Geometry: final body of the model. Coordinates: model frame, mm. Face numbers are marked on the shaded views. A direction names the side the tool comes from. Give positions to 0.01 mm unless a question says otherwise; leave off trailing zeros. Order: outer loops, then holes, each group sorted by start corner. A loop starts at its lowest first (then second) coordinate and runs counter-clockwise, first axis right, second up. Notation, with made-up numbers: (51, 65) -> (66, 65) arc R7 ccw to (66, 72) -> close; hole circle Ø1 at (-22.5, -19). An arc over 180 degrees is marked (long way). Write item = value, one per line.
```python
from build123d import *

# Parameters (mm, degrees)
SKETCH1_W                = 40
SKETCH1_H                = 48
BOSS_EXTRUDE1_DEPTH      = 4
BOSS_EXTRUDE2_DEPTH      = 11.15
BOSS_EXTRUDE2_DEPTH_BACK = 4
SKETCH5_W                = 40
SKETCH5_H                = 5.225
SKETCH5_W_2              = 18
SKETCH5_H_2              = 5
SKETCH5_H_3              = 6
FILLET1_DEPTH            = 40
SKETCH6_R                = 1.35
CUT_EXTRUDE4_DEPTH       = 58.214705278
CHAMFER2_SIZE            = 2
CHAMFER3_SIZE            = 3
CHAMFER3_SIZE2           = 1
CHAMFER4_SIZE            = 3
CHAMFER4_SIZE2           = 0.5
CUT_EXTRUDE6_DEPTH       = 10
CUT_EXTRUDE6_DEPTH_BACK  = 10
CUT_EXTRUDE8_REACH       = 66.292
SKETCH12_R               = 3
SKETCH13_R               = 1.5
CUT_EXTRUDE10_DEPTH      = 10.275
CUT_EXTRUDE7_DEPTH       = 1.25
CUT_EXTRUDE7_DEPTH_BACK  = 1.25
CHAMFER5_SIZE            = 5
CHAMFER5_SIZE2           = 3
CHAMFER6_SIZE            = 3
CHAMFER6_SIZE2           = 5
CUT_EXTRUDE12_DEPTH      = 46.535947422
CUT_EXTRUDE12_DEPTH_BACK = 46.535947422
SKETCH15_R               = 3.5


with BuildPart() as part:
    # Sketch1 → Boss-Extrude1 (new body)
    with BuildSketch(Plane.XY):
        with Locations((20, 14)):
            Rectangle(SKETCH1_W, SKETCH1_H)
    extrude(amount=BOSS_EXTRUDE1_DEPTH)

    # Sketch5 → Boss-Extrude2 (add, two sides: drawn at the far end of the back side and taken through both)
    with BuildSketch(Plane.XY.offset(4).offset(-BOSS_EXTRUDE2_DEPTH_BACK)):
        Polygon((0.9, 8.125), (0, 8.125), (0, 15.5), (40, 15.5), (40, 9), (28, 9), (27.357142857, 10.5), (11.081237185, 10.5), (9.763380042, 7.425), (8.800403155, 7.425), (8.500403155, 8.125), (7.531690021, 8.125), (7.231690021, 7.425), (6.221941609, 7.425), (5.921941609, 8.125), (5, 8.125), (4.7, 7.425), (3.7, 7.425), (3.4, 8.125), (2.5, 8.125), (2.2, 7.425), (1.2, 7.425), align=None)
        with Locations((20, 3.6125)):
            Rectangle(SKETCH5_W, SKETCH5_H)
        with Locations((20, -7.5)):
            Rectangle(SKETCH5_W_2, SKETCH5_H_2)
        with Locations((20, 35)):
            Rectangle(SKETCH5_W, SKETCH5_H_3)
    extrude(amount=BOSS_EXTRUDE2_DEPTH + BOSS_EXTRUDE2_DEPTH_BACK)

    # Fillet1: read off the stored shape, not the designer's step
    # Fillet1 outline → Fillet1 (add)
    with BuildSketch(Plane.YZ):
        with BuildLine():
            Line((32, 4), (32, 10))
            ThreePointArc((32, 10), (30.242640687, 5.757359313), (26, 4))
            Line((26, 4), (32, 4))
        make_face()
        with BuildLine():
            Line((1, 4), (1, 10))
            ThreePointArc((1, 10), (-0.757359313, 5.757359313), (-5, 4))
            Line((-5, 4), (1, 4))
        make_face()
    extrude(amount=FILLET1_DEPTH)

    # Sketch6 → Cut-Extrude4 (cut, through all)
    with BuildSketch(Plane.XY.offset(15.15)):
        with Locations((7.5, 35)):
            Circle(SKETCH6_R)
        with Locations((7.5, 12)):
            Circle(SKETCH6_R)
        with Locations((32.5, 35)):
            Circle(SKETCH6_R)
        with Locations((32.5, 12)):
            Circle(SKETCH6_R)
    extrude(amount=-CUT_EXTRUDE4_DEPTH, mode=Mode.SUBTRACT)

    # Chamfer2
    chamfer2_edges = [part.edges().sort_by_distance(p)[0] for p in [
        (40, 9, 9.575),
        (0, 15.5, 9.575),
        (40, 15.5, 9.575),
    ]]
    chamfer(chamfer2_edges, length=CHAMFER2_SIZE)

    # Chamfer3
    chamfer3_edges = [part.edges().sort_by_distance(p)[0] for p in [
        (4.2, 7.425, 15.15),
    ]]
    chamfer3_side = [part.faces().sort_by_distance(p)[0] for p in [
        (4.2, 7.425, 9.575),
    ]]
    chamfer(chamfer3_edges, length=CHAMFER3_SIZE, length2=CHAMFER3_SIZE2, reference=chamfer3_side[0])

    # Chamfer4
    chamfer4_edges = [part.edges().sort_by_distance(p)[0] for p in [
        (20, 6.225, 15.15),
    ]]
    chamfer4_side = [part.faces().sort_by_distance(p)[0] for p in [
        (20, 6.225, 9.575),
    ]]
    chamfer(chamfer4_edges, length=CHAMFER4_SIZE, length2=CHAMFER4_SIZE2, reference=chamfer4_side[0])

    # Sketch8 → Cut-Extrude6 (cut, two sides: drawn at the far end of the back side and taken through both)
    with BuildSketch(Plane(origin=(20, 0, 0), x_dir=(0, 0, -1), z_dir=(1, 0, 0)).offset(-CUT_EXTRUDE6_DEPTH_BACK)):
        with BuildLine():
            Line((-9, 34.1), (-18.820916768, 34.1))
            Line((-18.820916768, 34.1), (-18.820916768, 21.9))
            Line((-18.820916768, 21.9), (-9, 21.9))
            ThreePointArc((-9, 21.9), (-2.9, 28), (-9, 34.1))
        make_face()
        with BuildLine():
            Line((-18.820916768, -10.472551988), (-18.820916768, -3.194214037))
            Line((-18.820916768, -3.194214037), (-13.313351365, 2.313351365))
            ThreePointArc((-13.313351365, 2.313351365), (-3.364334852, 0.334368937), (-9, -8.1))
            Line((-9, -8.1), (-9, -10.472551988))
            Line((-9, -10.472551988), (-18.820916768, -10.472551988))
        make_face()
    extrude(amount=CUT_EXTRUDE6_DEPTH + CUT_EXTRUDE6_DEPTH_BACK, mode=Mode.SUBTRACT)

    # Cut-Extrude8: up to this face of the body (flat: up to its plane)
    cut_extrude8_end = Plane(part.part.faces().sort_by_distance((20, 15.5, 9.575))[0])
    # Sketch12 → Cut-Extrude8 (cut, up to the picked face)
    with BuildSketch(Plane(origin=(0, 38, 0), x_dir=(1, 0, 0), z_dir=(0, 1, 0)), mode=Mode.PRIVATE) as cut_extrude8_sk1:
        with Locations(Location((15.4, -9, 0), (0, 0, 270))):
            Circle(SKETCH12_R)
    cut_extrude8_tool1 = split(extrude(cut_extrude8_sk1.sketch, amount=-CUT_EXTRUDE8_REACH, mode=Mode.PRIVATE), bisect_by=cut_extrude8_end, keep=Keep.BOTH, mode=Mode.PRIVATE)
    add(cut_extrude8_tool1.solids().sort_by(Axis((15.4, 38, 9), (0, -1, 0)))[0], mode=Mode.SUBTRACT)

    # Sketch13 → Cut-Extrude10 (cut)
    with BuildSketch(Plane(origin=(0, 15.5, 0), x_dir=(1, 0, 0), z_dir=(0, 1, 0))):
        with Locations(Location((15.4, -9, 0), (0, 0, 180))):
            Circle(SKETCH13_R)
    extrude(amount=-CUT_EXTRUDE10_DEPTH, mode=Mode.SUBTRACT)

    # Sketch9 → Cut-Extrude7 (cut, two sides: drawn at the far end of the back side and taken through both)
    with BuildSketch(Plane.XZ.offset(-13).offset(-CUT_EXTRUDE7_DEPTH_BACK)):
        Polygon((12.5, 16.815347994), (18.3, 16.815347994), (18.3, 7.325684219), (15.4, 5.651368439), (12.5, 7.325684219), align=None)
    extrude(amount=CUT_EXTRUDE7_DEPTH + CUT_EXTRUDE7_DEPTH_BACK, mode=Mode.SUBTRACT)

    # Chamfer5
    chamfer5_edges = [part.edges().sort_by_distance(p)[0] for p in [
        (0, 38, 7.575),
    ]]
    chamfer5_side = [part.faces().sort_by_distance(p)[0] for p in [
        (20.225127502, 38, 7.505259415),
    ]]
    chamfer(chamfer5_edges, length=CHAMFER5_SIZE, length2=CHAMFER5_SIZE2, reference=chamfer5_side[0])

    # Chamfer6
    chamfer6_edges = [part.edges().sort_by_distance(p)[0] for p in [
        (40, 38, 7.575),
    ]]
    chamfer6_side = [part.faces().sort_by_distance(p)[0] for p in [
        (40, 5.721658913, 8.075),
    ]]
    chamfer(chamfer6_edges, length=CHAMFER6_SIZE, length2=CHAMFER6_SIZE2, reference=chamfer6_side[0])

    # Sketch15 → Cut-Extrude12 (cut, two sides: drawn at the far end of the back side and taken through both)
    with BuildSketch(Plane(origin=(20, 0, 0), x_dir=(0, 0, -1), z_dir=(1, 0, 0)).offset(-CUT_EXTRUDE12_DEPTH_BACK)):
        with Locations((-9, -2)):
            Circle(SKETCH15_R)
    extrude(amount=CUT_EXTRUDE12_DEPTH + CUT_EXTRUDE12_DEPTH_BACK, mode=Mode.SUBTRACT)


solid = part.part
```
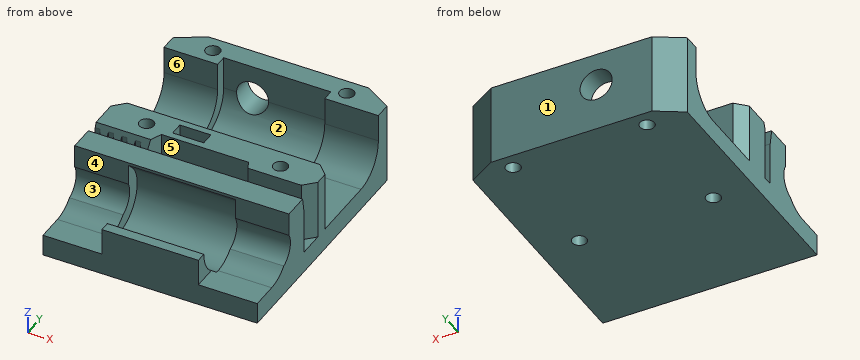
1) Reachability of the marked faces 4, 5 and 6 from +Z, -Z, +X, -X, +Y, -Y: full face, straight path, thin tool, end or side. Return the list, or none.
Check sheet entries:
face_4 = +Z, +X, -X, -Y
face_5 = +Z
face_6 = +Z, +X, -X
2) Section query B-B (y = -3). Output: boundary loops of the cut face in (x, z).
Check sheet entries:
outline = (0, 0) -> (40, 0) -> (40, 4.34) -> (30, 4.34) -> (30, 2.98) -> (10, 2.98) -> (10, 4.34) -> (0, 4.34) -> close
3) First-contact query: P1, Ø4, axis at x = 15, y = 18.5, coming from the +Z side; P2, Ø1, axis at x = 0.5, z = 7.5, coming from the -Y side; P3, Ø5.5, axis at x = 33, z = 12, coming from the -Y side; P4, Ø10, axis at x = 8, y = 6.5, coming from the +Z side. Flat tips, straight axial feed; report the tip coordinate or a pass-through.
Check sheet entries:
P1 = 4
P2 = 0.87
P3 = 1
P4 = 15.15
4) Section query A-A (x = 32.5). Output: boundary loops of the cut face in (y, z) (3 decimals).
Check sheet entries:
outline = (-10, 0) -> (10.65, 0) -> (10.65, 15.15) -> (9, 15.15) -> (9, 4) -> (6.225, 4) -> (6.225, 12.15) -> (5.725, 15.15) -> (1, 15.15) -> (1, 10.803) arc R3.5 cw to (-0.805, 5.71) arc R6 cw to (-5, 4) -> (-10, 4) -> close; (13.35, 0) -> (33.65, 0) -> (33.65, 15.15) -> (32, 15.15) -> (32, 10) arc R6 cw to (26, 4) -> (15.5, 4) -> (15.5, 15.15) -> (13.35, 15.15) -> close; (36.35, 0) -> (38, 0) -> (38, 15.15) -> (36.35, 15.15) -> close
5) Mould query, pull axis Z, two halves, no side actions, for the marked faces 1, 2 and 3. Classes: +Z half, -Z half, draft (parallel to the pull), parting line (faces both ways), or undercut.
Check sheet entries:
face_1 = draft
face_2 = +Z half
face_3 = undercut
6) Line query: line 1 (Y direction, x = 7.5, z = 1.75); line 2 (X direction, y = 31.5, z = 7); line 3 (Z direction, x = 15.4, y = 15). Output: solid intervals per line, ascending. Write a range as from..to.
Check sheet entries:
line_1 = -10..10.65, 13.35..33.65, 36.35..38
line_2 = 0..10, 30..40
line_3 = 0..7.5, 10.5..15.15
